```python
from build123d import *


with BuildPart() as part:
    # Croquis1 → Revolución1 (revolve)
    with BuildSketch(Plane(origin=(0, 0, 0), x_dir=(1, 0, 0), z_dir=(0, 1, 0)), mode=Mode.PRIVATE) as revoluci_n1_sk:
        with BuildLine():
            Line((0, 7.5), (2, 7.5))
            Line((2, 7.5), (2, 9))
            Line((2, 9), (0, 9))
            Line((0, 9), (0, 8.75))
            Line((0, 8.75), (1.375452526, 8.495838133))
            ThreePointArc((1.375452526, 8.495838133), (1.580025529, 8.25), (1.375452526, 8.004161867))
            Line((1.375452526, 8.004161867), (0, 7.75))
            Line((0, 7.75), (0, 7.5))
        make_face()
    revolve(revoluci_n1_sk.sketch.rotate(Axis((0, 0, 0), (1, 0, 0)), 180), axis=Axis((0, 0, 0), (1, 0, 0)))


solid = part.part
```
Model file for the job. Use its own axes, mm. Round coordinates to 2 decimals unless told otherwise and drop trailing zeros. Loops run counter-clockwise (first coordinate to the right, second up) from the corner with the lowest first, then second, coordinate; pieces in that order, holes last. Notation, with made-up numbers: M 71,-11.5 L 130,-11.5 A27 cw 130,16.5 Z; hole C -13,50.25 d3. An arc over 180 degrees is marked long. Put each result on its own line as item: value. Start each with the question number.
Item 1: Drill centre lines: line 1 along Y through (x, z) = (1.35, 0.5); line 2 along Y through (x, z) = (0.5, -5.25); line 3 along Z through (x, y) = (0.65, -3.5). Where is each one in solid material? Low to high.
Item 2: Cut at C-C (x = 0.9). List the corners of the cut face in (y, z).
Item 3: Mould opens along Y. For faces 1 (the face through (0.986, -6.083, -6.633)), 2 (the face through (2, -7.4, 2)), 3 (the face through (1.014, -6.324, 4.032)) say: released by +Y, released by -Y, zero draft, split by the parting line, or undercut.
Item 4: Drop a flat-ended pin along its axis: P1, Ø6, axis at y = 1.5, z = -4, coming from the -X side. Give the stop position or say it passes through.
Item 5: Cut at A-A (z = 0). List the corners of the cut face in (x, y).
Answer block:
1. line 1: -8.99 to -8.49, -7.98 to -7.48, 7.48 to 7.98, 8.49 to 8.99
1. line 2: -7.31 to -6.88, -5.83 to -5.36, 5.36 to 5.83, 6.88 to 7.31
1. line 3: -8.29 to -7.89, -7.05 to -6.63, 6.63 to 7.05, 7.89 to 8.29
2. outline: C 0,0 d18; C 0,0 d15.83; hole C 0,0 d17.17; hole C 0,0 d15
3. face 1: split by the parting line
3. face 2: zero draft
3. face 3: undercut
4. P1: through
5. outline: M 0,-9 L 2,-9 L 2,-7.5 L 0,-7.5 L 0,-7.75 L 1.38,-8 A0.25 cw 1.38,-8.5 L 0,-8.75 Z; M 0,7.5 L 2,7.5 L 2,9 L 0,9 L 0,8.75 L 1.38,8.5 A0.25 cw 1.38,8 L 0,7.75 Z
